Could you check a few things on this model? Use its own coordinates, in mm. Face numbers are marked on the shaded views. A direction names the side the tool comes from. Coordinates: 2 decimals unless noted, no trailing zeros. Write each loop counter-clockwise with the first axis right and the second up, starting at its lowest first coordinate (ties: lowest second). Pieces come first, ordered by that corner, then holes. Notation, with made-up numbers: (21, 74) - (77, 74) arc R22 cw to (77, 111) - close; hole circle Ø7 at (25, 65.5). An arc over 180 degrees is marked (long way). Answer as a JSON object with one key per item and string values. Group by question number.
1) If we section it at A-A (y = 203): Write out the boundary of the cut face in (x, z).
2) Please list where these lines run through material, in increasing order: line 1 along Y through (x, z) = (457, 14) (3 decimals); line 2 along Z through (x, y) = (458.5, 101); line 3 along Z through (x, y) = (-20, 141.5).
3) On a 3-axis mill with a long thin cutter (end or side, diameter ignored), from which of +Z, -Z, +X, -X, +Y, -Y can I reach the whole of each face in a straight line? I mean the marked faces 4 and 5. Say none if no direction works.
4) If we section it at B-B (x = 690.5): Write out the boundary of the cut face in (y, z) (3 decimals).
5) Will these pins go through, and if not, where does the flat tip stop? pin 1 Ø10 at (y, z) = (23.5, 288) entering from +X; pin 2 Ø10 at (x, y) = (745, -77) entering from +Z; pin 3 Ø5 at (y, z) = (123.5, 297) entering from +X.
6) If we section it at C-C (z = 312): Write out the boundary of the cut face in (x, y) (3 decimals).
7) We'd pull the mould along Z, two halves only. Please class the marked faces 1, 2 and 3: released by +Z, released by -Z, zero draft, split by the parting line, or undercut.
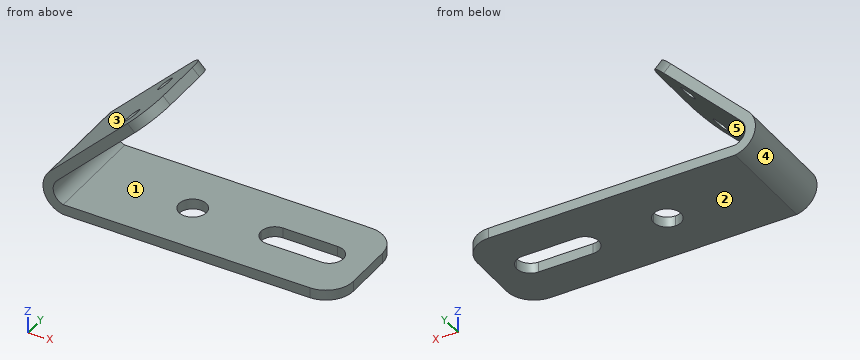
```python
from build123d import *

# Parameters (mm, degrees)
F0_W     = 1270
F0_H     = 48.26
F1_DEPTH = 241.935
F3_DEPTH = 254
F5_DEPTH = 127
F6_R     = 38.1
F7_DEPTH = 101.6
F8_R     = 127


with BuildPart() as f1:
    # F0 (on Front) → F1 (new body, symmetric)
    with BuildSketch(Plane.XZ):
        with Locations((635, 24.13)):
            Rectangle(F0_W, F0_H)
        with BuildLine():
            ThreePointArc((-61.369352, 189.382638), (-88.660331, 75.904336), (0, 0))
            Line((0, 0), (0, 48.26))
            ThreePointArc((0, 48.26), (-44.826748, 94.123068), (-27.992452, 156.005738))
            Line((-27.992452, 156.005738), (421.020354, 605.018544))
            Line((421.020354, 605.018544), (387.643454, 638.395444))
            Line((387.643454, 638.395444), (-61.369352, 189.382638))
        make_face()
    extrude(amount=F1_DEPTH, both=True)

    # F2 (on face) → F3 (cut)
    with BuildSketch(Plane(origin=(0, 0, 0), x_dir=(1, 0, 0), z_dir=(0, 0, -1))):
        with BuildLine():
            ThreePointArc((1092.2, -63.5), (1137.101281, -44.901281), (1155.7, 0))
            ThreePointArc((1155.7, 0), (1137.101281, 44.901281), (1092.2, 63.5))
            Line((1092.2, 63.5), (838.2, 63.5))
            ThreePointArc((838.2, 63.5), (793.298719, 44.901281), (774.7, 0))
            ThreePointArc((774.7, 0), (793.298719, -44.901281), (838.2, -63.5))
            Line((838.2, -63.5), (1092.2, -63.5))
        make_face()
    extrude(amount=-F3_DEPTH, mode=Mode.SUBTRACT)

    # F4 (on face) → F5 (cut)
    with BuildSketch(Plane(origin=(0, 0, 0), x_dir=(1, 0, 0), z_dir=(0, 0, -1))):
        with BuildLine():
            ThreePointArc((520.7, 0), (502.101281, 44.901281), (457.2, 63.5))
            ThreePointArc((457.2, 63.5), (412.298719, -44.901281), (520.7, 0))
        make_face()
    extrude(amount=-F5_DEPTH, mode=Mode.SUBTRACT)

    # F6 (on face) → F7 (cut)
    with BuildSketch(Plane(origin=(-125.375995, 0, 125.375995), x_dir=(0, -1, 0), z_dir=(-0.707107, 0, 0.707107))):
        with BuildLine():
            ThreePointArc((-127.761006, 573.119062), (-154.701775, 508.078294), (-89.661006, 535.019062))
            ThreePointArc((-89.661006, 535.019062), (-100.820238, 561.959831), (-127.761006, 573.119062))
        make_face()
        with Locations((127.761006, 535.019062)):
            Circle(F6_R)
    extrude(amount=-F7_DEPTH, mode=Mode.SUBTRACT)

    # F8
    f8_edges = [f1.edges().sort_by_distance(p)[0] for p in [
        (404.331904, 241.935, 621.706994),
        (404.331904, -241.935, 621.706994),
        (1270, -241.935, 24.13),
        (1270, 241.935, 24.13),
    ]]
    fillet(f8_edges, radius=F8_R)


solid = f1.part
```
Here are the results:
{
 "1": {"outline": "(-61.37, 189.38) arc R111.76 ccw to (0, 0) - (1234.51, 0) - (1234.51, 48.26) - (0, 48.26) arc R64.56 cw to (-27.99, 156.01) - (395.92, 579.92) - (362.55, 613.3) - close"},
 "2": {"line 1": "y = -241.935 to -63.5, 63.5 to 241.935", "line 2": "z = 0 to 48.26", "line 3": "z = 5.13 to 57.92, 164 to 230.75"},
 "3": {"face 4": "-X, +Y, -Y", "face 5": "+X, +Y, -Y"},
 "4": {"outline": "(-241.935, 0) - (241.935, 0) - (241.935, 48.26) - (-241.935, 48.26) - close"},
 "5": {"pin 1": "stops at x = 109", "pin 2": "stops at z = 48.26", "pin 3": "stops at x = 115.5"},
 "6": {"outline": "(61.248, -241.935) - (128.002, -241.935) - (128.002, 241.935) - (61.248, 241.935) - close"},
 "7": {"face 1": "undercut", "face 2": "released by -Z", "face 3": "released by +Z"}
}
